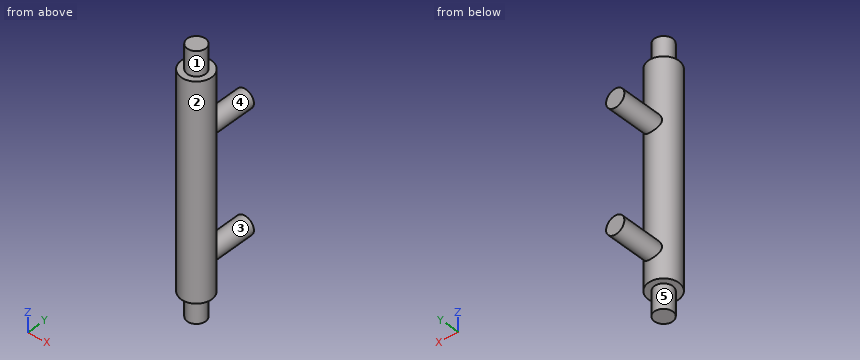
Autodesk Inventor part; units mm, degrees
ref_plane "Work Plane1" through (0, 18, 0) normal (0, 1, 0) x (-1, 0, 0)
ref_plane "YZ Plane" through (0, 0, 0) normal (1, 0, 0) x (0, 1, 0)
ref_plane "XY Plane" through (0, 0, 0) normal (0, 0, 1) x (1, 0, 0)
sketch "Sketch1" plane through (0, 0, 0) normal (0, 0, 1) x (1, 0, 0)
  circle A0 centre (0, 0) radius 5
  dimension "d0" = 10
extrude "Extrusion1" add sketch "Sketch1" along normal blind 70
sketch "Sketch2" plane through (0, 0, 70) normal (0, 0, 1) x (1, 0, 0)
  circle A0 centre (0, 0) radius 3
  dimension "d3" = 6
extrude "Extrusion2" add sketch "Sketch2" along normal blind 8
sketch "Sketch3" plane through (0, 0, 0) normal (0, 0, -1) x (-1, 0, 0)
  circle A0 centre (0, 0) radius 3
  circle A1 centre (0, 0) radius 3
  dimension "d6" = 6
extrude "Extrusion3" add sketch "Sketch3" along normal blind 8
ref_plane "Work Plane1" through (0, 18, 0) normal (0, 1, 0) x (-1, 0, 0)
sketch "Sketch4" plane through (0, 18, 0) normal (0, 1, 0) x (-1, 0, 0)
  circle A0 centre (0, 10) radius 3
  circle A1 centre (0, 50) radius 3
  line L0 (5, 0) -> (5, 70)
  line L1 (5, 35) -> (17.3974, 35) construction
  point P0 (0, 0)
  dimension "d10" = 6
  dimension "d11" = 6
  dimension "d12" = 40
  dimension "d13" = 10
extrude "Extrusion4" add sketch "Sketch4" against normal up to surface
properties part number "verbindung2"
Design review of the part built by this model. Coordinates are the model's own, in mm. Face numbers are marked on the shaded views. A direction names the side the tool comes from. Give positions to 0.01 mm unless a question says otherwise; leave off trailing zeros. Order: outer loops, then holes, each group sorted by start corner. A loop starts at its lowest first (then second) coordinate and runs counter-clockwise, first axis right, second up. Notation, with made-up numbers: (-13, 67) - (19, 67) arc R28 cw to (19, 95) - close; hole circle Ø11 at (-33, 65.5). An arc over 180 degrees is marked (long way). Use CSV: the item, a comma, the result in double quotes. Start each with the question number.
Q1. Draft analysis for pull direction Z (two halves, no side actions). For the marked faces 4 and 5, state which applies: pulls with the +Z half, pulls with the -Z half, needs draft (parallel to the pull), parting line crosses it, or undercut.
Q2. For P1, Ø12, axis at y = 10.5, z = 14, coming from the +X side; P2, Ø4, axis at x = -3, z = 37, coming from the +Y side; P3, Ø12, axis at y = 15.5, z = 65.5, coming from the -X side; P4, Ø2, axis at x = 0.5, y = 12.5, coming from the -Z side, all flat-tipped, find the tip position at first contact; note any pin that passes through.
Q3. Take a section at A-A (y = 0). State the section outline as (x, z) points.
Q4. Machinability: for the marked faces 1, 2 and 3, which of the approach directions +Z, -Z, +X, -X, +Y, -Y give a long, thin tool a straight path to every point of the face, cutting with its end or side? Answer none if there is none.
Q5. Take a section at C-C (z = 39.5). State the section outline as (x, y) points.
Q6. For line 1 (Z direction, x = -3.75, y = -0.75); line 2 (Z direction, x = -2.5, y = 11.75); line 3 (Y direction, x = -4, z = 14), list the stretches that pass through material, from the lowest coordinate up.
Q7. Take a section at B-B (x = 0). State the section outline as (y, z) points.
Q8. Take a section at D-D (z = 10). State the section outline as (x, y) points, and give its area (3 significant figures).
Calculated:
1,face 4,"undercut"
1,face 5,"needs draft"
2,P1,"stops at x = 3"
2,P2,"stops at y = 4.9"
2,P3,"passes through"
2,P4,"stops at z = 7"
3,outline,"(-5, 0) - (-3, 0) - (-3, -8) - (3, -8) - (3, 0) - (5, 0) - (5, 70) - (3, 70) - (3, 78) - (-3, 78) - (-3, 70) - (-5, 70) - close"
4,face 1,"+Z"
4,face 2,"none"
4,face 3,"+Y"
5,outline,"circle Ø10 at (0, 0)"
6,line 1,"z = 0 to 70"
6,line 2,"z = 8.34 to 11.66, 48.34 to 51.66"
6,line 3,"y = -3 to 3"
7,outline,"(-5, 0) - (-3, 0) - (-3, -8) - (3, -8) - (3, 0) - (5, 0) - (5, 7) - (18, 7) - (18, 13) - (5, 13) - (5, 47) - (18, 47) - (18, 53) - (5, 53) - (5, 70) - (3, 70) - (3, 78) - (-3, 78) - (-3, 70) - (-5, 70) - close"
8,outline,"(-3, 4) arc R5 ccw (long way) to (3, 4) - (3, 18) - (-3, 18) - close"
8,area,"158 mm²"
